Source: three-view drawing plus pictorial views. Frame: mm from the lowest corner of the part. Give positions to 0.01 mm unless a question says otherwise; leave off trailing zeros. Order: outer loops, then holes, each group sorted by start corner. A loop starts at its lowest first (then second) coordinate and runs counter-clockwise, first axis right, second up. Notation, with made-up numbers: (40.25, 81) -> (71.25, 81) arc R29 ccw to (71.25, 113) -> close; hole circle Ø8 at (-29.75, 88.5). An arc over 180 degrees is marked (long way). Use a Markdown table: item, result. Add a question column.
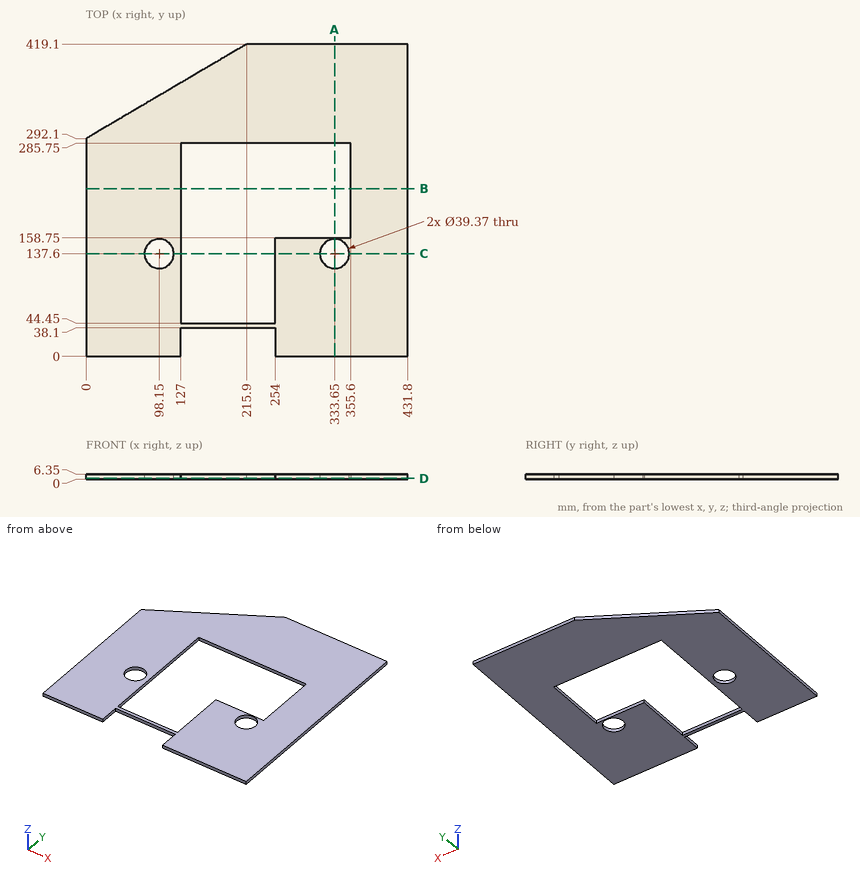
Q1. First-contact query: pin 1 (3 mm diameter, centred on y = 120.5, z = 2.5, fed in from -X); pin 2 (2 mm diameter, centred on x = 212, z = 3, fed in from +Y); pin 3 (3 mm diameter, centred on x = 206, z = 3.5, fed in from -Y); pin 4 (3 mm diameter, centred on x = 195, z = 3.5, fed in from +Y). Flat tips, straight axial feed; report the tip coordinate or a pass-through.
Q2. Section query B-B (y = 225). Return loops of the section in (x, z), plus the area to 3 significant figures.
Q3. Section query C-C (y = 137.6). Return loops of the section in (x, z) (3 decimals), plus the area to 3 significant figures.
Q4. Section query A-A (x = 333.65). Return loops of the section in (y, z) (3 decimals), plus the area to 3 significant figures.
Q5. Ray query, line 1 (X direction, y = 204.5, z = 5.75); line 2 (Y direction, x = 333.65, z = 2) (3 decimals); line 3 (Y direction, x = 297, z = 0.75). Return the intervals inside material, ascending.
Q6. Section query D-D (z = 1). Return loops of the section in (x, y) (3 decimals), plus the area to 3 significant figures.
Solution:
| question | item | result |
|---|---|---|
| 1 | pin 1 | stops at x = 0 |
| 1 | pin 2 | stops at y = 417.39 |
| 1 | pin 3 | stops at y = 38.1 |
| 1 | pin 4 | stops at y = 407.69 |
| 2 | outline | (0, 0) -> (127, 0) -> (127, 6.35) -> (0, 6.35) -> close; (355.6, 0) -> (431.8, 0) -> (431.8, 6.35) -> (355.6, 6.35) -> close |
| 2 | area | 1,290 mm² |
| 3 | outline | (0, 0) -> (78.465, 0) -> (78.465, 6.35) -> (0, 6.35) -> close; (117.835, 0) -> (127, 0) -> (127, 6.35) -> (117.835, 6.35) -> close; (254, 0) -> (313.965, 0) -> (313.965, 6.35) -> (254, 6.35) -> close; (353.335, 0) -> (431.8, 0) -> (431.8, 6.35) -> (353.335, 6.35) -> close |
| 3 | area | 1,440 mm² |
| 4 | outline | (0, 0) -> (117.915, 0) -> (117.915, 6.35) -> (0, 6.35) -> close; (157.285, 0) -> (158.75, 0) -> (158.75, 6.35) -> (157.285, 6.35) -> close; (285.75, 0) -> (419.1, 0) -> (419.1, 6.35) -> (285.75, 6.35) -> close |
| 4 | area | 1,600 mm² |
| 5 | line 1 | x = 0 to 127, 355.6 to 431.8 |
| 5 | line 2 | y = 0 to 117.915, 157.285 to 158.75, 285.75 to 419.1 |
| 5 | line 3 | y = 0 to 158.75, 285.75 to 419.1 |
| 6 | outline | (0, 0) -> (127, 0) -> (127, 38.1) -> (254, 38.1) -> (254, 0) -> (431.8, 0) -> (431.8, 419.1) -> (215.9, 419.1) -> (0, 292.1) -> close; hole circle Ø39.37 at (98.15, 137.6); hole (127, 44.45) -> (254, 44.45) -> (254, 158.75) -> (355.6, 158.75) -> (355.6, 285.75) -> (127, 285.75) -> close; hole circle Ø39.37 at (333.65, 137.6) |
| 6 | area | 116,000 mm² |
